Can you work these out from the drawing? Everything is in mm from the part's minimum corner. A direction names the side the tool comes from. Give positions to 0.01 mm unless a question says otherwise; leave off trailing zeros. Order: outer loops, then holes, each group sorted by start corner. A loop starts at its lowest first (then second) coordinate and runs counter-clockwise, first axis right, second up. Notation, with made-up numbers: M 17,77 L 39,77 A29 cw 39,99 Z; hole C 32,7 d1. An arc over 180 degrees is marked long. Answer as a JSON object with one key per item and string values.
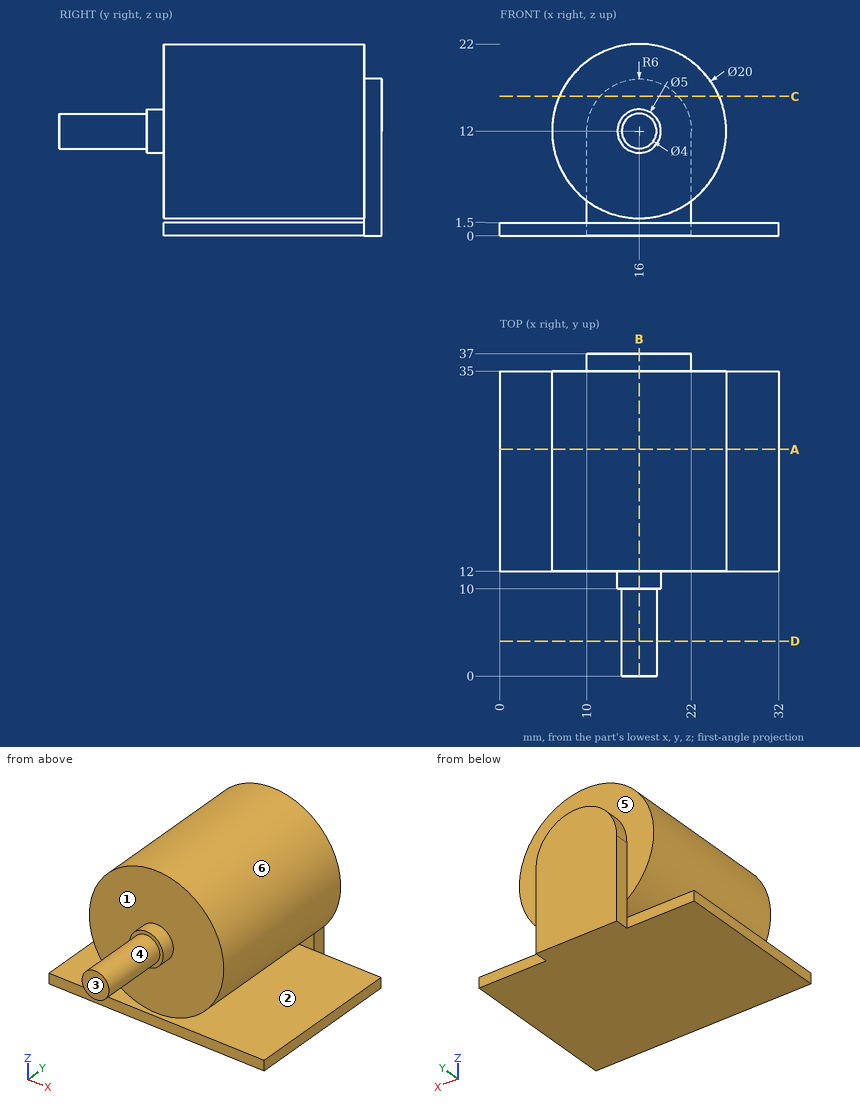
1) I need wall thicknesses on L1, parallel to Z at x = 16, y = 13; L2, parallel to Y at x = 19.5, z = 16.25; L3, parallel to Z at x = 1, y = 14. Which ranges of each line are inside material? Lowest first, please.
Results found:
{"L1": "z = 0 to 1.5, 2 to 22", "L2": "y = 12 to 37", "L3": "z = 0 to 1.5"}
2) I want a section at C-C on z = 16. Write out the boundary of the cut face in (x, y), and give its area (3 significant figures).
Results found:
{"outline": "M 6.83,12 L 25.17,12 L 25.17,35 L 20.47,35 L 20.47,37 L 11.53,37 L 11.53,35 L 6.83,35 Z", "area": "439 mm²"}
3) I want a section at D-D on y = 4. Write out the boundary of the cut face in (x, z), and give its area (3 significant figures).
Results found:
{"outline": "C 16,12 d4", "area": "12.6 mm²"}
4) I want a section at B-B on x = 16. Write out the boundary of the cut face in (y, z).
Results found:
{"outline": "M 0,10 L 10,10 L 10,9.5 L 12,9.5 L 12,2 L 35,2 L 35,1.5 L 12,1.5 L 12,0 L 37,0 L 37,18 L 35,18 L 35,22 L 12,22 L 12,14.5 L 10,14.5 L 10,14 L 0,14 Z"}
5) I want a section at A-A on y = 26. Write out the boundary of the cut face in (x, z).
Results found:
{"outline": "M 0,0 L 32,0 L 32,1.5 L 0,1.5 Z; C 16,12 d20"}
6) For the marked faces 1, 2 and 3, which set-ups out of +Z, -Z, +X, -X, +Y, -Y let a thin tool reach every point of the face, with its end or its side?
Results found:
{"face 1": "-Y", "face 2": "+X, -X, -Y", "face 3": "+Z, -Z, +X, -X, -Y"}
7) I'm going to push flat-ended pins straight in: pin 1 Ø8 at (x, y) = (18.5, 6.5) entering from -Z; pin 2 Ø3 at (y, z) = (19, 12) entering from -X; pin 3 Ø10 at (y, z) = (19.5, 12) entering from +X. Where does each tip first touch, or does it pass through?
Results found:
{"pin 1": "stops at z = 9.56", "pin 2": "stops at x = 6", "pin 3": "stops at x = 26"}
8) Thinking about a two-plate mould opening in Z: for the marked faces 4, 5 and 6, which applies, pulls with the +Z half, pulls with the -Z half, needs draft (parallel to the pull), parting line crosses it, or undercut?
Results found:
{"face 4": "parting line crosses it", "face 5": "needs draft", "face 6": "undercut"}
